Read the model definition and answer for the solid it produces. Units are mm, in the model's axes. Give positions to 0.01 mm unless a question says otherwise; leave off trailing zeros. Order: outer loops, then holes, each group sorted by start corner. A loop starts at its lowest first (then second) coordinate and runs counter-clockwise, first axis right, second up. Notation, with made-up numbers: (7, 63.5) - (25, 63.5) arc R11 cw to (25, 74.5) - close; hole circle Ø9 at (19, 85.5). An arc over 180 degrees is marked (long way). Write each question's results on one line, items separated by ' | '. Start each with the question number.
Q1. Find section C-C on y = 9. Give the vertices of the cut face in (x, z), and give its area (3 significant figures).
Q2. Find section A-A on x = -34.5. Give the vertices of the cut face in (y, z), and give its area (3 significant figures).
Q3. Find the intervals of material crossed by line 1 along X through (y, z) = (48, 1.25); line 2 along X through (y, z) = (19, 1.25); line 3 along Y through (x, z) = (-24, 0.5), in increasing order. Write a range as from..to.
Q4. Find section D-D on x = -20. Give the vertices of the cut face in (y, z), and give its area (3 significant figures).
Q5. Flat-ended cylindrical pins translate along their axes: P1, Ø1.8, axis at x = -63.448, y = 71.664, coming from the -Z side; P2, Ø2.5, axis at x = -2.799, y = 3.556, coming from the +Z side; P3, Ø0.6, axis at y = 76, z = 3.5, coming from the +X side. Find the tip coordinate at first contact, or state that the pin passes through.
Q6. Find section B-B on y = 21.5. Give the vertices of the cut face in (x, z).
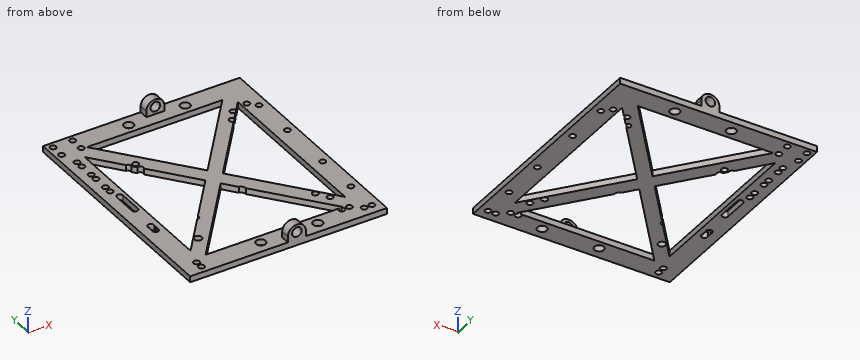
from build123d import *

# Parameters (mm, degrees)
SKETCH3_W            = 65.532
SKETCH3_H            = 78.232
SKETCH3_R            = 1
SKETCH3_R_2          = 1.25
SKETCH3_R_3          = 1.6
BOSS_EXTRUDE10_DEPTH = 2
SKETCH5_R            = 1.6
BOSS_EXTRUDE11_DEPTH = 3


with BuildPart() as part:
    # Sketch3 → Boss-Extrude10 (new body)
    with BuildSketch(Plane.XY):
        with Locations((-32.766, 39.116)):
            Rectangle(SKETCH3_W, SKETCH3_H)
        with Locations((-60.198, 2.535)):
            Circle(SKETCH3_R, mode=Mode.SUBTRACT)
        with Locations((-60.198, 5.075)):
            Circle(SKETCH3_R, mode=Mode.SUBTRACT)
        with Locations((-53.34, 15.24)):
            Circle(SKETCH3_R_2, mode=Mode.SUBTRACT)
        with Locations((-39.450944, 4.064)):
            Circle(SKETCH3_R_3, mode=Mode.SUBTRACT)
        with BuildLine():
            ThreePointArc((-60.547487864, 25.781), (-60.378588258, 25.483259443), (-60.32, 25.146))
            ThreePointArc((-60.32, 25.146), (-61.657259443, 24.204588258), (-62.092512136, 25.781))
            ThreePointArc((-62.092512136, 25.781), (-62.32, 26.416), (-62.092512136, 27.051))
            ThreePointArc((-62.092512136, 27.051), (-61.657259443, 28.627411742), (-60.32, 27.686))
            ThreePointArc((-60.32, 27.686), (-60.378588258, 27.348740557), (-60.547487864, 27.051))
            ThreePointArc((-60.547487864, 27.051), (-60.378588258, 26.753259443), (-60.32, 26.416))
            ThreePointArc((-60.32, 26.416), (-60.378588258, 26.078740557), (-60.547487864, 25.781))
        make_face(mode=Mode.SUBTRACT)
        with BuildLine():
            Line((-11.628420455, 7), (-56.019094707, 7))
            Line((-56.019094707, 7), (-33.112109743, 35.552384115))
            Line((-33.112109743, 35.552384115), (-29.697720228, 31.296522373))
            ThreePointArc((-29.697720228, 31.296522373), (-28.738744364, 30.752879791), (-28.359, 29.718))
            ThreePointArc((-28.359, 29.718), (-28.359594089, 29.67440261), (-28.361375915, 29.630837597))
            Line((-28.361375915, 29.630837597), (-10.205124779, 7))
            Line((-10.205124779, 7), (-10.773355545, 7))
            ThreePointArc((-10.773355545, 7), (-10.356041134, 6.631008199), (-10.200888, 6.096))
            ThreePointArc((-10.200888, 6.096), (-11.735896199, 5.251153134), (-11.628420455, 7))
        make_face(mode=Mode.SUBTRACT)
        with Locations((-20.574, 3.890944)):
            Circle(SKETCH3_R_3, mode=Mode.SUBTRACT)
        with Locations((-8.700888, 6.096)):
            Circle(SKETCH3_R, mode=Mode.SUBTRACT)
        with Locations((-5.339, 3.556)):
            Circle(SKETCH3_R, mode=Mode.SUBTRACT)
        with Locations((-2.799, 3.556)):
            Circle(SKETCH3_R, mode=Mode.SUBTRACT)
        with Locations((-10.668, 13.208)):
            Circle(SKETCH3_R, mode=Mode.SUBTRACT)
        with Locations((-13.213, 17.018)):
            Circle(SKETCH3_R, mode=Mode.SUBTRACT)
        with Locations((-2.794, 14.728)):
            Circle(SKETCH3_R, mode=Mode.SUBTRACT)
        with Locations((-2.794, 29.718)):
            Circle(SKETCH3_R, mode=Mode.SUBTRACT)
        with BuildLine():
            ThreePointArc((-61.706, 45.116), (-60.706, 46.116), (-59.706, 45.116))
            Line((-59.706, 45.116), (-59.706, 37.116))
            ThreePointArc((-59.706, 37.116), (-60.706, 36.116), (-61.706, 37.116))
            Line((-61.706, 37.116), (-61.706, 45.116))
        make_face(mode=Mode.SUBTRACT)
        with Locations((-61.722, 48.629)):
            Circle(SKETCH3_R, mode=Mode.SUBTRACT)
        with Locations((-61.722, 51.169)):
            Circle(SKETCH3_R, mode=Mode.SUBTRACT)
        with Locations((-61.722, 56.129)):
            Circle(SKETCH3_R, mode=Mode.SUBTRACT)
        with Locations((-61.722, 58.669)):
            Circle(SKETCH3_R, mode=Mode.SUBTRACT)
        with BuildLine():
            Line((-58.532, 10.995023961), (-58.532, 67.236976039))
            Line((-58.532, 67.236976039), (-50.821827001, 57.626640091))
            ThreePointArc((-50.821827001, 57.626640091), (-50.014999166, 57.252778474), (-49.824952048, 56.384086494))
            Line((-49.824952048, 56.384086494), (-48.700366603, 54.982348306))
            ThreePointArc((-48.700366603, 54.982348306), (-47.474999166, 54.712778474), (-47.477503777, 53.458112393))
            Line((-47.477503777, 53.458112393), (-35.971124779, 39.116))
            Line((-35.971124779, 39.116), (-47.320258494, 24.969885803))
            ThreePointArc((-47.320258494, 24.969885803), (-47.275179837, 24.801577784), (-47.26, 24.628))
            ThreePointArc((-47.26, 24.628), (-47.600460693, 23.876329925), (-48.390015804, 23.636488078))
            Line((-48.390015804, 23.636488078), (-58.532, 10.995023961))
        make_face(mode=Mode.SUBTRACT)
        with Locations((-48.255, 56.627)):
            Circle(SKETCH3_R, mode=Mode.SUBTRACT)
        Polygon((-32.766, 43.111023961), (-55.326875221, 71.232), (-10.205124779, 71.232), align=None, mode=Mode.SUBTRACT)
        with Locations((-61.722, 63.629)):
            Circle(SKETCH3_R, mode=Mode.SUBTRACT)
        with Locations((-61.722, 66.169)):
            Circle(SKETCH3_R, mode=Mode.SUBTRACT)
        with Locations((-63.448, 71.664)):
            Circle(SKETCH3_R, mode=Mode.SUBTRACT)
        with Locations((-63.448, 76.164)):
            Circle(SKETCH3_R, mode=Mode.SUBTRACT)
        with Locations((-56.948, 71.664)):
            Circle(SKETCH3_R, mode=Mode.SUBTRACT)
        with Locations((-56.948, 76.164)):
            Circle(SKETCH3_R, mode=Mode.SUBTRACT)
        with Locations((-39.37, 74.422)):
            Circle(SKETCH3_R_3, mode=Mode.SUBTRACT)
        with BuildLine():
            Line((-9.668009055, 64.774255485), (-7, 68.099792192))
            Line((-7, 68.099792192), (-7, 10.995023961))
            Line((-7, 10.995023961), (-29.906984964, 39.547408077))
            Line((-29.906984964, 39.547408077), (-13.321002101, 60.220986655))
            ThreePointArc((-13.321002101, 60.220986655), (-13.983000834, 61.839778474), (-12.259188179, 61.544483353))
            Line((-12.259188179, 61.544483353), (-10.455353631, 63.792870775))
            ThreePointArc((-10.455353631, 63.792870775), (-11.448000834, 65.395778474), (-9.668009055, 64.774255485))
        make_face(mode=Mode.SUBTRACT)
        with Locations((-2.794, 48.514)):
            Circle(SKETCH3_R, mode=Mode.SUBTRACT)
        with Locations((-20.574, 74.422)):
            Circle(SKETCH3_R_3, mode=Mode.SUBTRACT)
        with Locations((-2.794, 63.504)):
            Circle(SKETCH3_R, mode=Mode.SUBTRACT)
        with Locations((-5.309112, 66.04)):
            Circle(SKETCH3_R, mode=Mode.SUBTRACT)
    extrude(amount=BOSS_EXTRUDE10_DEPTH)

    # Sketch5 → Boss-Extrude11 (add)
    with BuildSketch(Plane.XZ):
        with BuildLine():
            Line((-33.014, 2), (-27.014, 2))
            Line((-27.014, 2), (-27.014, 4))
            ThreePointArc((-27.014, 4), (-30.014, 7), (-33.014, 4))
            Line((-33.014, 4), (-33.014, 2))
        make_face()
        with Locations(Location((-30.014, 4.5, 0), (0, 0, 270))):
            Circle(SKETCH5_R, mode=Mode.SUBTRACT)
    boss_extrude11 = extrude(amount=-BOSS_EXTRUDE11_DEPTH)

    # Mirror1: Boss-Extrude11 across plane
    add(boss_extrude11.mirror(Plane.ZX.offset(39.116)))


solid = part.part
Working result:
1) outline: (-65.53, 0) - (-54.41, 0) - (-54.41, 2) - (-65.53, 2) - close; (-11.81, 0) - (0, 0) - (0, 2) - (-11.81, 2) - close | area: 45.9 mm²
2) outline: (0, 0) - (7, 0) - (7, 2) - (0, 2) - close; (33.82, 0) - (45.27, 0) - (45.27, 2) - (33.82, 2) - close; (71.23, 0) - (78.23, 0) - (78.23, 2) - (71.23, 2) - close | area: 50.9 mm²
3) line 1: -65.53..-62.5, -60.94..-58.53, -43.1..-36.69, -28.84..-23.13, -7..-3.65, -1.94..0 | line 2: -65.53..-58.53, -52.11..-46.39, -19.83..-13.42, -7..0 | line 3: 0..7, 24.19..32.18, 46.91..54.04, 71.23..78.23
4) outline: (0, 0) - (2.4, 0) - (2.4, 2) - (0, 2) - close; (5.38, 0) - (7, 0) - (7, 2) - (5.38, 2) - close; (19.21, 0) - (27.2, 0) - (27.2, 2) - (19.21, 2) - close; (51.9, 0) - (59.02, 0) - (59.02, 2) - (51.9, 2) - close; (71.23, 0) - (72.93, 0) - (72.93, 2) - (71.23, 2) - close; (75.92, 0) - (78.23, 0) - (78.23, 2) - (75.92, 2) - close | area: 46.3 mm²
5) P1: through | P2: z = 2 | P3: x = -27.01
6) outline: (-65.53, 0) - (-58.53, 0) - (-58.53, 2) - (-65.53, 2) - close; (-50.1, 0) - (-44.39, 0) - (-44.39, 2) - (-50.1, 2) - close; (-21.84, 0) - (-15.43, 0) - (-15.43, 2) - (-21.84, 2) - close; (-7, 0) - (0, 0) - (0, 2) - (-7, 2) - close
